Model file for the job. Use its own axes, mm. Face numbers are marked on the shaded views. A direction names the side the tool comes from. Round coordinates to 2 decimals unless told otherwise and drop trailing zeros. Order: outer loops, then holes, each group sorted by start corner. A loop starts at its lowest first (then second) coordinate and runs counter-clockwise, first axis right, second up. Notation, with made-up numbers: M 38.25,39 L 94.25,39 A28 cw 94.25,60 Z; hole C 3.25,-8.75 d5. An arc over 180 degrees is marked long. Return JSON: item names as keys, results as strings. Group by question number.
Item 1: Pin check, flat tips, straight feed: pin 1 Ø12 at (x, z) = (-20, -7) entering from +Y; pin 2 Ø3 at (x, y) = (28.5, 2.5) entering from +Z; pin 3 Ø11 at (x, z) = (35, 9) entering from +Y; pin 4 Ø17.5 at (x, z) = (32, -6.5) entering from +Y. Stop position of each tip, or through.
Item 2: Slice it at A-A on y = 0. Write the cut outline in (x, z).
Item 3: Slice it at B-B on x = 35. Write the cut outline in (y, z), then the cut area to 3 significant figures.
Item 4: Slice it at C-C on z = 12. Write the cut outline in (x, y), then the cut area to 3 significant figures.
Item 5: Pull direction Z, two halves, no side cores. Call the marked faces 3, 4, 5 and 6: pulls with the +Z half, pulls with the -Z half, needs draft (parallel to the pull), parting line crosses it, or undercut.
Item 6: Slice it at D-D on x = 0. Write the cut outline in (y, z), then the cut area to 3 significant figures.
Item 7: Which spindle directions (+Z, -Z, +X, -X, +Y, -Y) get a long thin tool onto all of the face, cutting with end or side? Do the marked faces 1 and 2. Say none if no direction does.
Item 8: Probe line 1 along Z through (x, y) = (-35, -10.5); line 2 along Z through (x, y) = (-32, 14.5); line 3 along Y through (x, z) = (6, 5). List the from-to ranges inside material, lowest first.
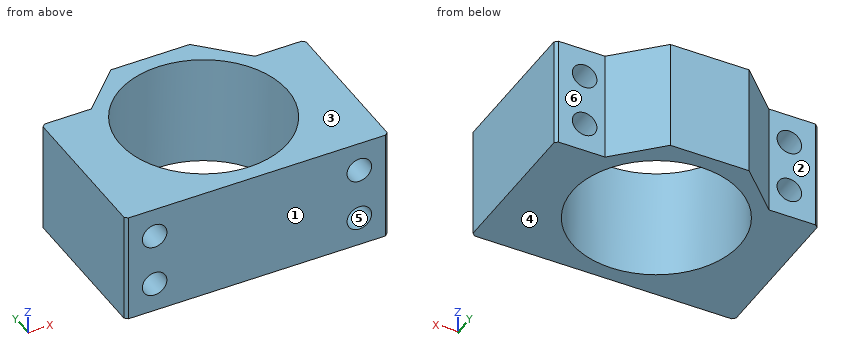
from build123d import *

# Parameters (mm, degrees)
SKETCH1_W            = 90
SKETCH1_H            = 68
SKETCH1_R            = 28.65
BOSS_EXTRUDE1_DEPTH  = 19
M8_CLEARANCE_HOLE1_D = 8.4
CUT_EXTRUDE2_DEPTH   = 39
CHAMFER1_SIZE        = 1


with BuildPart() as part:
    # Sketch1 → Boss-Extrude1 (new body, symmetric)
    with BuildSketch(Plane.XY):
        Rectangle(SKETCH1_W, SKETCH1_H)
        Circle(SKETCH1_R, mode=Mode.SUBTRACT)
    extrude(amount=BOSS_EXTRUDE1_DEPTH, both=True)

    # M8 Clearance Hole1 (through all)
    with Locations(Plane(origin=(0, 34, 0), x_dir=(1, 0, 0), z_dir=(0, 1, 0))):
        with Locations((-35, 9), (-35, -9), (35, -9), (35, 9)):
            Hole(M8_CLEARANCE_HOLE1_D / 2)

    # Sketch3 → Cut-Extrude2 (cut, through all)
    with BuildSketch(Plane.XY.offset(19)):
        Polygon((-45, 19.5), (-28, 19.5), (-13.5, 34), (-45, 34), align=None)
        Polygon((45, 19.5), (28, 19.5), (13.5, 34), (45, 34), align=None)
    extrude(amount=-CUT_EXTRUDE2_DEPTH, mode=Mode.SUBTRACT)

    # Chamfer1
    chamfer1_edges = [part.edges().sort_by_distance(p)[0] for p in [
        (-45, 19.5, 0),
        (45, 19.5, 0),
        (45, -34, 0),
        (-45, -34, 0),
    ]]
    chamfer(chamfer1_edges, length=CHAMFER1_SIZE)


solid = part.part
Output values:
{
 "1": {"pin 1": "y = 33.5", "pin 2": "z = 19", "pin 3": "y = 19.5", "pin 4": "y = 24.25"},
 "2": {"outline": "M -45,-19 L -28.65,-19 L -28.65,19 L -45,19 Z; M 28.65,-19 L 45,-19 L 45,19 L 28.65,19 Z; hole C -35,-9 d8.4; hole C -35,9 d8.4; hole C 35,-9 d8.4; hole C 35,9 d8.4"},
 "3": {"outline": "M -34,-19 L 19.5,-19 L 19.5,-13.2 L -34,-13.2 Z; M -34,-4.8 L 19.5,-4.8 L 19.5,4.8 L -34,4.8 Z; M -34,13.2 L 19.5,13.2 L 19.5,19 L -34,19 Z", "area": "1,130 mm²"},
 "4": {"outline": "M -45,-33 L -44,-34 L -37.94,-34 L -37.94,19.5 L -44,19.5 L -45,18.5 Z; M -32.06,-34 L 32.06,-34 L 32.06,19.5 L 28,19.5 L 13.5,34 L -13.5,34 L -28,19.5 L -32.06,19.5 Z; M 37.94,-34 L 44,-34 L 45,-33 L 45,18.5 L 44,19.5 L 37.94,19.5 Z; hole C 0,0 d57.3", "area": "2,210 mm²"},
 "5": {"face 3": "pulls with the +Z half", "face 4": "pulls with the -Z half", "face 5": "undercut", "face 6": "needs draft"},
 "6": {"outline": "M -34,-19 L -28.65,-19 L -28.65,19 L -34,19 Z; M 28.65,-19 L 34,-19 L 34,19 L 28.65,19 Z", "area": "407 mm²"},
 "7": {"face 1": "+Z, -Z, +X, -X, -Y", "face 2": "+Z, -Z, -X, +Y"},
 "8": {"line 1": "-19 to -13.2, -4.8 to 4.8, 13.2 to 19", "line 2": "-19 to -11.94, -6.06 to 6.06, 11.94 to 19", "line 3": "-34 to -28.01, 28.01 to 34"}
}
